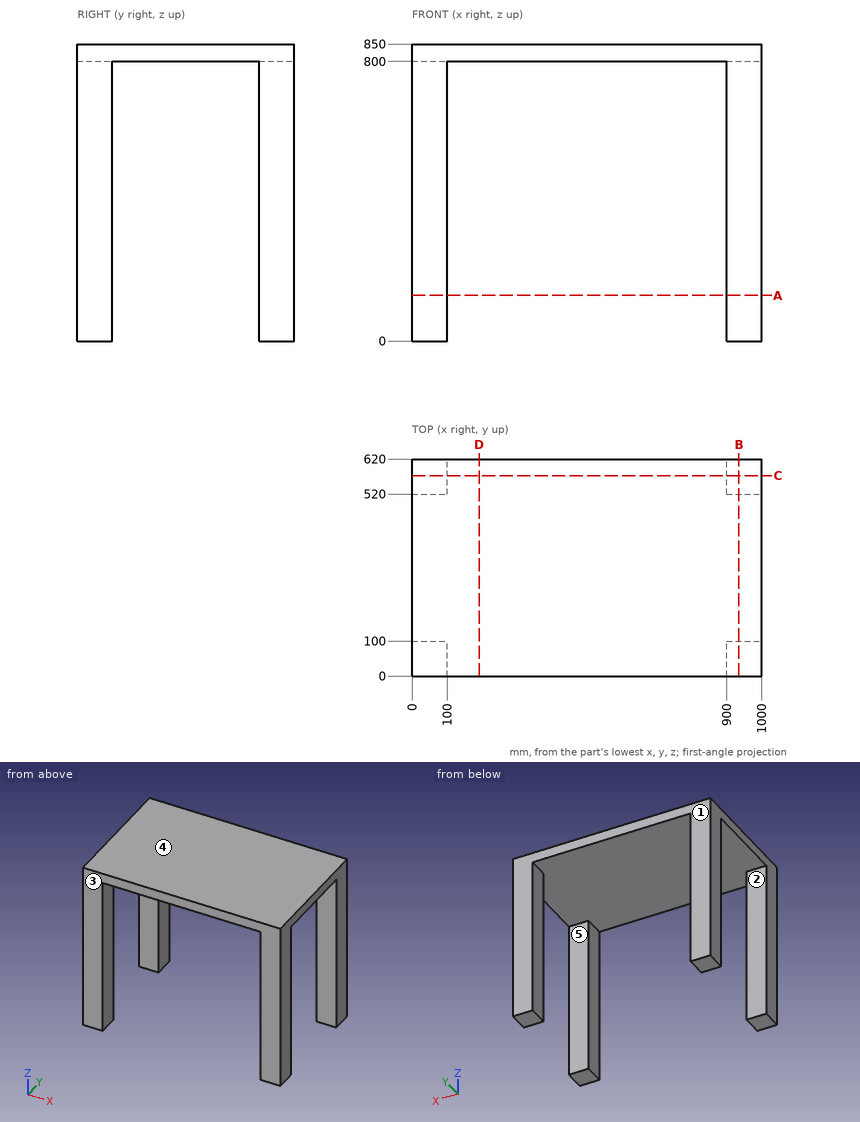
For this review, use the dimensioned drawing (mm, ordinates from the lowest corner) and the shaded views. A direction names the side the tool comes from. Coordinates: 2 decimals unless noted, no trailing zeros. Order: outer loops, then holes, each group sorted by start corner. A loop starts at its lowest first (then second) coordinate and runs counter-clockwise, first axis right, second up. Notation, with made-up numbers: M 32.25,58.25 L 85.25,58.25 A4 cw 85.25,65.25 Z; hole C -1.5,-30.5 d5. An arc over 180 degrees is marked long. Answer as a JSON object with one key per item and string values. Group by question number.
1) Wall thickness on L1, parallel to X at y = 587.5, z = 376; L2, parallel to Y at x = 75.5, z = 479.5; L3, parallel to Z at x = 356.5, y = 47: over which ranges is each line inside the solid? List them lowest first.
2) Add section B-B, the plane x = 934.5. Write out the cut boundary in (y, z).
3) Add section D-D, the plane x = 192. Write out the cut boundary in (y, z).
4) Mouldability with a two-part tool opening along Y and no side actions: class the marked faces 3, 4 and 5 as pulls with the +Y half, pulls with the -Y half, needs draft (parallel to the pull), parting line crosses it, or undercut.
5) Tool access review of the marked faces 1 and 2: name each direction out of +Z, -Z, +X, -X, +Y, -Y from which nothing blocks a thin tool from reaching the whole face with its end or side.
6) Add section A-A, the plane z = 131. Write out the cut boundary in (x, y), then the cut area to 3 significant figures.
7) Add section C-C, the plane y = 573. Write out the cut boundary in (x, z), then the cut area to 3 significant figures.
Computed values:
{
 "1": {"L1": "x = 0 to 100, 900 to 1000", "L2": "y = 0 to 100, 520 to 620", "L3": "z = 800 to 850"},
 "2": {"outline": "M 0,0 L 100,0 L 100,800 L 520,800 L 520,0 L 620,0 L 620,850 L 0,850 Z"},
 "3": {"outline": "M 0,800 L 620,800 L 620,850 L 0,850 Z"},
 "4": {"face 3": "pulls with the -Y half", "face 4": "needs draft", "face 5": "undercut"},
 "5": {"face 1": "+Z, -Z, +X, -X, +Y", "face 2": "-Z, +X, -X"},
 "6": {"outline": "M 0,0 L 100,0 L 100,100 L 0,100 Z; M 0,520 L 100,520 L 100,620 L 0,620 Z; M 900,0 L 1000,0 L 1000,100 L 900,100 Z; M 900,520 L 1000,520 L 1000,620 L 900,620 Z", "area": "40,000 mm^2"},
 "7": {"outline": "M 0,0 L 100,0 L 100,800 L 900,800 L 900,0 L 1000,0 L 1000,850 L 0,850 Z", "area": "210,000 mm^2"}
}
